Model file for the job. Use its own axes, mm. Give positions to 0.01 mm unless a question says otherwise; leave off trailing zeros. Write each loop counter-clockwise with the first axis right and the second up, starting at its lowest first coordinate (ties: lowest second). Pieces come first, ordered by that corner, then holes. Notation, with made-up numbers: M 43.5,62 L 90.5,62 A21 cw 90.5,101 Z; hole C 1,60 d6. An arc over 180 degrees is marked long. Answer as a JSON object with one key per item and string values. Group by question number.
```python
from build123d import *

# Parameters (mm, degrees)
F0_R     = 1.5875
F1_DEPTH = 2.38125


# Not quite as in the source:
# - a length typed as a fraction of an inch, garbled in the dataset ("3 / 203.2 mm" for 3/8 in), is restored


with BuildPart() as f1:
    # F0 (on Top) → F1 (new body)
    with BuildSketch(Plane.XY):
        with BuildLine():
            Line((0, -12.7), (0, 0))
            Line((0, 0), (0, 12.7))
            Line((0, 12.7), (-32.55645, 12.7))
            ThreePointArc((-32.55645, 12.7), (-45.25645, 0), (-32.55645, -12.7))
            Line((-32.55645, -12.7), (0, -12.7))
        make_face()
        with BuildLine():
            ThreePointArc((-30.96895, -6.35), (-33.6789820151, -7.4725320151), (-32.55645, -4.7625))
            ThreePointArc((-32.55645, -4.7625), (-31.4339179849, -5.2274679849), (-30.96895, -6.35))
        make_face(mode=Mode.SUBTRACT)
        with Locations((-38.90645, 0)):
            Circle(F0_R, mode=Mode.SUBTRACT)
        with BuildLine():
            ThreePointArc((-32.55645, 3.96875), (-29.7501199622, 2.8063300378), (-28.5877, 0))
            ThreePointArc((-28.5877, 0), (-29.7501199622, -2.8063300378), (-32.55645, -3.96875))
            ThreePointArc((-32.55645, -3.96875), (-35.3627800378, -2.8063300378), (-36.5252, 0))
            ThreePointArc((-36.5252, 0), (-35.3627800378, 2.8063300378), (-32.55645, 3.96875))
        make_face(mode=Mode.SUBTRACT)
        with BuildLine():
            ThreePointArc((-24.61895, 0), (-26.20645, -1.5875), (-27.79395, 0))
            ThreePointArc((-27.79395, 0), (-26.20645, 1.5875), (-24.61895, 0))
        make_face(mode=Mode.SUBTRACT)
        with BuildLine():
            ThreePointArc((-30.96895, 6.35), (-31.4339179849, 5.2274679849), (-32.55645, 4.7625))
            ThreePointArc((-32.55645, 4.7625), (-33.6789820151, 7.4725320151), (-30.96895, 6.35))
        make_face(mode=Mode.SUBTRACT)
        with BuildLine():
            Line((0, 12.7), (0, 0))
            Line((0, 0), (0, -12.7))
            Line((0, -12.7), (32.54375, -12.7))
            ThreePointArc((32.54375, -12.7), (45.24375, 0), (32.54375, 12.7))
            Line((32.54375, 12.7), (0, 12.7))
        make_face()
        with Locations((32.55645, -6.35)):
            Circle(F0_R, mode=Mode.SUBTRACT)
        with BuildLine():
            ThreePointArc((27.79395, 0), (26.20645, -1.5875), (24.61895, 0))
            ThreePointArc((24.61895, 0), (26.20645, 1.5875), (27.79395, 0))
        make_face(mode=Mode.SUBTRACT)
        with BuildLine():
            ThreePointArc((36.5125, 0), (32.54375, -3.96875), (28.575, 0))
            ThreePointArc((28.575, 0), (32.54375, 3.96875), (36.5125, 0))
        make_face(mode=Mode.SUBTRACT)
        with Locations((38.90645, 0)):
            Circle(F0_R, mode=Mode.SUBTRACT)
        with Locations((32.55645, 6.35)):
            Circle(F0_R, mode=Mode.SUBTRACT)
    extrude(amount=F1_DEPTH)


solid = f1.part
```
Q1. Slice it at A-A, the plane z = 1.9. Count the separate pieces of the cut face and the enclosed holes in it, then the cut area to 3 significant figures.
Q2. Slice it at B-B, the plane x = 39. Write the cut outline in (y, z).
Q3. Two-plate mould, pull along Y, no slides. Class faces 1 (the cylindrical face through (-45.253, 0.279, 1.174)), 2 (the flat face through (-1, 0, 0)), 3 (the cylindrical face through (40.42, 0.48, 1.17)): +Y half, -Y half, draft (parallel to the pull), parting line (faces both ways), or undercut.
Q4. Slice it at D-D, the plane y = -2.75. Write the cut outline in (x, z).
Q5. Slice it at C-C, the plane y = 2.5. Write the cut outline in (x, z).
Q6. Drop a flat-ended pin along its axis: P1, Ø2.5, axis at x = -38.91, y = 0, coming from the +Z side. Give the stop position or say it passes through.
Q7. Wall check: L1, parallel to X at y = 6.75, z = 1.65; L2, parallel to X at y = -5.25, z = 1.15; L3, parallel to Y at x = -34, z = 1.8. Give the ranges that are in metal, low to high.
Solved:
{
 "1": {"separate pieces": "1", "enclosed holes": "10", "area": "2,000 mm²"},
 "2": {"outline": "M -10.94,0 L -1.58,0 L -1.58,2.38 L -10.94,2.38 Z; M 1.58,0 L 10.94,0 L 10.94,2.38 L 1.58,2.38 Z"},
 "3": {"face 1": "parting line", "face 2": "draft", "face 3": "undercut"},
 "4": {"outline": "M -44.96,0 L -35.42,0 L -35.42,2.38 L -44.96,2.38 Z; M -29.69,0 L 29.68,0 L 29.68,2.38 L -29.69,2.38 Z; M 35.41,0 L 44.94,0 L 44.94,2.38 L 35.41,2.38 Z"},
 "5": {"outline": "M -45.01,0 L -35.64,0 L -35.64,2.38 L -45.01,2.38 Z; M -29.47,0 L 29.46,0 L 29.46,2.38 L -29.47,2.38 Z; M 35.63,0 L 45,0 L 45,2.38 L 35.63,2.38 Z"},
 "6": {"P1": "passes through"},
 "7": {"L1": "x = -43.31 to -34.09, -31.02 to 31.02, 34.09 to 43.3", "L2": "x = -44.12 to -33.7, -31.41 to 31.41, 33.7 to 44.11", "L3": "y = -12.62 to -7.01, -5.69 to -3.7, 3.7 to 5.69, 7.01 to 12.62"}
}
